Part model, mm, in its own coordinate system. Round coordinates to 2 decimals unless told otherwise and drop trailing zeros. Use a Markdown table: item, result. Add a question column.
Item 1: Probe line 1 (Z direction, x = 0, y = 27); line 2 (Z direction, x = -8.75, y = 28.5); line 3 (X direction, y = 23.6, z = 0). List the from-to ranges inside material, lowest first. Write a range as [from, to].
Item 2: Two-plate mould, pull along Z, no slides. Class faces 1 (the face through (-6, 22.225, 3)), 2 (the face through (-3.86, 23.79, 5.04)): pulls with the +Z half, pulls with the -Z half, needs draft (parallel to the pull), parting line crosses it, or undercut.
Item 3: Flat gauge pins, fed straight in: pin 1 (4 mm diameter, centred on x = -2.5, z = -3, fed in from +Y); pin 2 (8 mm diameter, centred on y = 27.5, z = 4.5, fed in from +X); pin 3 (10 mm diameter, centred on x = -3.5, y = 33.5, fed in from -Z). Where does each tip first touch, or does it go through?
```python
from build123d import *

# Parameters (mm, degrees)
CUT_EXTRUDE1_REACH             = 47.963
SKETCH2_W                      = 34.925
SKETCH2_H                      = 22.225
CUT_EXTRUDE1_DIRECTION_2_REACH = 47.963
CUT_EXTRUDE2_DEPTH             = 9.525
CIRPATTERN1_COUNT              = 3
SKETCH6_R                      = 6.35
CUT_EXTRUDE3_DEPTH             = 3.175


with BuildPart() as part:
    # Sketch1 → Revolve1 (revolve)
    with BuildSketch(Plane.XY):
        with BuildLine():
            Line((0, 41.275), (0, 0))
            Line((0, 0), (7.5, 0))
            ThreePointArc((7.5, 0), (12.485619708, 5.484310547), (14.299969698, 12.670561319))
            ThreePointArc((14.299969698, 12.670561319), (14.3, 12.7), (14.299969698, 12.729438681))
            ThreePointArc((14.299969698, 12.729438681), (12.201631467, 26.047427638), (6.1595, 38.1))
            ThreePointArc((6.1595, 38.1), (3.464825582, 40.434546629), (0, 41.275))
        make_face()
    revolve(axis=Axis((0, 0, 0), (0, 1, 0)))

    # Sketch2 → Cut-Extrude1 (cut, up to next)
    with BuildSketch(Plane(origin=(0, 0, 0), x_dir=(0, 0, -1), z_dir=(1, 0, 0)), mode=Mode.PRIVATE) as cut_extrude1_sk1:
        with Locations((0, 11.1125)):
            Rectangle(SKETCH2_W, SKETCH2_H)
    cut_extrude1_tool1 = extrude(cut_extrude1_sk1.sketch, amount=-CUT_EXTRUDE1_REACH, mode=Mode.PRIVATE) & part.part
    add(cut_extrude1_tool1.solids().sort_by_distance((0, 11.1125, 0))[0], mode=Mode.SUBTRACT)

    # Sketch2 → Cut-Extrude1 direction 2 (cut, up to next)
    with BuildSketch(Plane(origin=(0, 0, 0), x_dir=(0, 0, -1), z_dir=(1, 0, 0)), mode=Mode.PRIVATE) as cut_extrude1_direction_2_sk1:
        with Locations((0, 11.1125)):
            Rectangle(SKETCH2_W, SKETCH2_H)
    cut_extrude1_direction_2_tool1 = extrude(cut_extrude1_direction_2_sk1.sketch, amount=CUT_EXTRUDE1_DIRECTION_2_REACH, mode=Mode.PRIVATE) & part.part
    add(cut_extrude1_direction_2_tool1.solids().sort_by_distance((0, 11.1125, 0))[0], mode=Mode.SUBTRACT)

    # Sketch3 → Cut-Extrude2 (cut)
    with BuildSketch(Plane.XZ.offset(-22.225)):
        with BuildLine():
            Line((-2.434829201, -1.7526), (2.434829201, -1.7526))
            ThreePointArc((2.434829201, -1.7526), (0, 3), (-2.434829201, -1.7526))
        make_face()
    extrude(amount=-CUT_EXTRUDE2_DEPTH, mode=Mode.SUBTRACT)

    # Cut-Sweep1: sweep along a path in Sketch4
    with BuildLine(Plane.XY) as cut_sweep1_path:
        Line((-6.35, 41.275), (-6.35, 39.7002))
        ThreePointArc((-6.35, 39.7002), (-6.599150778, 37.96819754), (-7.326398315, 36.376651231))
        ThreePointArc((-7.326398315, 36.376651231), (-10.906399133, 29.561182531), (-13.240375425, 22.225))
    # Sketch5 → Cut-Sweep1 (sweep, cut)
    with BuildSketch(Plane.XZ.offset(-22.225)):
        with BuildLine():
            ThreePointArc((-13.04083059, 2.290039063), (-12.065, 0), (-13.04083059, -2.290039063))
            ThreePointArc((-13.04083059, -2.290039063), (-13.240375425, 0), (-13.04083059, 2.290039063))
        make_face()
    cut_sweep1 = sweep(path=cut_sweep1_path.line, mode=Mode.SUBTRACT)

    # CirPattern1: Cut-Sweep1 ×3 about axis
    cirpattern1_axis = Axis((0, 42.243264125, 0), (0, -1, 0))
    for i in range(1, CIRPATTERN1_COUNT):
        add(cut_sweep1.rotate(cirpattern1_axis, i * 360 / CIRPATTERN1_COUNT), mode=Mode.SUBTRACT)

    # Sketch6 → Cut-Extrude3 (cut)
    with BuildSketch(Plane.XZ.offset(-22.225)):
        with Locations(Location((0, 0, 0), (0, 0, 270))):
            Circle(SKETCH6_R)
    extrude(amount=-CUT_EXTRUDE3_DEPTH, mode=Mode.SUBTRACT)


solid = part.part
```
A:
| question | item | result |
|---|---|---|
| 1 | line 1 | z = [-11.88, -1.75], [3, 11.88] |
| 1 | line 2 | z = [-7.2, 7.2] |
| 1 | line 3 | x = [-11.72, -6.35], [6.35, 12.91] |
| 2 | face 1 | needs draft |
| 2 | face 2 | undercut |
| 3 | pin 1 | stops at y = 41.03 |
| 3 | pin 2 | stops at x = 12.55 |
| 3 | pin 3 | stops at z = -11.07 |
